from build123d import *

# Parameters (mm, degrees)
BOSS_EXTRUDE1_DEPTH       = 25
F_4_0MM_DOWEL_HOLE1_D     = 4
F_4_0MM_DOWEL_HOLE1_DEPTH = 17.29
F_4_0MM_DOWEL_HOLE1_TIP   = 1.201721238


with BuildPart() as part:
    # Sketch1 → Boss-Extrude1 (new body)
    with BuildSketch(Plane(origin=(0, 0, 0), x_dir=(0, 0, -1), z_dir=(1, 0, 0))):
        with BuildLine():
            Line((10, 84), (-20, 84))
            ThreePointArc((-20, 84), (-21, 85), (-20, 86))
            Line((-20, 86), (10, 86))
            ThreePointArc((10, 86), (96, 0), (10, -86))
            ThreePointArc((10, -86), (9, -85), (10, -84))
            ThreePointArc((10, -84), (94, 0), (10, 84))
        make_face()
    extrude(amount=BOSS_EXTRUDE1_DEPTH)

    # Ø4.0mm Dowel Hole1
    with Locations(Plane(origin=(0, 86, 0), x_dir=(1, 0, 0), z_dir=(0, 1, 0))):
        with Locations((12.5, -14), (12.5, 4)):
            Hole(F_4_0MM_DOWEL_HOLE1_D / 2, depth=F_4_0MM_DOWEL_HOLE1_DEPTH)
            with Locations((0, 0, -(F_4_0MM_DOWEL_HOLE1_DEPTH + F_4_0MM_DOWEL_HOLE1_TIP / 2))):  # 118° drill point
                Cone(0, F_4_0MM_DOWEL_HOLE1_D / 2, F_4_0MM_DOWEL_HOLE1_TIP, mode=Mode.SUBTRACT)


solid = part.part
Verification items for the finished model (mm, model axes). Give positions to 0.01 mm unless a question says otherwise; leave off trailing zeros. Write each loop counter-clockwise with the first axis right and the second up, starting at its lowest first coordinate (ties: lowest second). Pieces come first, ordered by that corner, then holes. Notation, with made-up numbers: (-13.75, 50) - (16.25, 50) arc R12 ccw to (16.25, 55) - close; hole circle Ø7 at (-19.5, 4.25). An arc over 180 degrees is marked (long way). Answer as CSV lines item,"result". Start each with the question number.
1. Sectioned sample at C-C (z = -15). Record the boundary of the cut face in (x, y).
2. Sectioned sample at D-D (y = -11). Record the boundary of the cut face in (x, z).
3. Sectioned sample at A-A (z = 14). Record the boundary of the cut face in (x, y).
4. Sectioned sample at B-B (x = 12.5). Record the boundary of the cut face in (y, z), then the cut area to 3 significant figures.
5. Depth check by flat-ended pin: pin 1 (10 mm diameter, centred on x = 17.5, y = 23, fed in from +Z); pin 2 (4 mm diameter, centred on x = 22.5, y = -20, fed in from -Z); pin 3 (6 mm diameter, centred on x = 16.5, z = -22, fed in from +Y). Enter the tip coordinate at first touch or a pass-through.
6. Thickness scan on line 1 (Y direction, x = 6.75, z = 0); line 2 (Y direction, x = 8, z = -75); line 3 (X direction, y = 84.55, z = 14). Record the ranges inside material, lowest first.
7. Draft check along Z on faces 1 (the face through (12, 86, 5)), 2 (the face through (12.32, -1.85, -93.98)), 3 (the face through (13.974, 84.986, 12.648)). Enter one of: pulls with the +Z half, pulls with the -Z half, needs draft (parallel to the pull), parting line crosses it, or undercut.
Derived:
1,outline,"(0, -85.85) - (25, -85.85) - (25, -83.85) - (0, -83.85) - close; (0, 83.85) - (25, 83.85) - (25, 85.85) - (0, 85.85) - close"
2,outline,"(0, -95.29) - (25, -95.29) - (25, -93.28) - (0, -93.28) - close"
3,outline,"(0, 84) - (10.5, 84) - (10.5, 86) - (0, 86) - close; (14.5, 84) - (25, 84) - (25, 86) - (14.5, 86) - close"
4,outline,"(-86, -10) arc R86 ccw to (86, -10) - (86, -6) - (84, -6) - (84, -10) arc R84 cw to (-84, -10) arc R1 ccw to start; (84, -2) - (86, -2) - (86, 12) - (84, 12) - close; (84, 16) - (86, 16) - (86, 20) arc R1 ccw to (84, 20) - close"
4,area,"581 mm²"
5,pin 1,"z = -89.2"
5,pin 2,"z = -94.1"
5,pin 3,"y = 85.53"
6,line 1,"84 to 86"
6,line 2,"-56.31 to -53.21, 53.21 to 56.31"
6,line 3,"0 to 10.5, 14.5 to 25"
7,face 1,"needs draft"
7,face 2,"pulls with the +Z half"
7,face 3,"undercut"
